Could you check a few things on this model? Use its own coordinates, in mm. Face numbers are marked on the shaded views. A direction names the side the tool comes from. Give positions to 0.01 mm unless a question says otherwise; leave off trailing zeros. Order: outer loops, then holes, each group sorted by start corner. A loop starts at its lowest first (then second) coordinate and runs counter-clockwise, first axis right, second up. Notation, with made-up numbers: M 53,87.5 L 100,87.5 A30 ccw 100,111.5 Z; hole C 29,52.5 d5. An arc over 180 degrees is marked long. Answer in a Markdown table with one row per item. Add a question column.
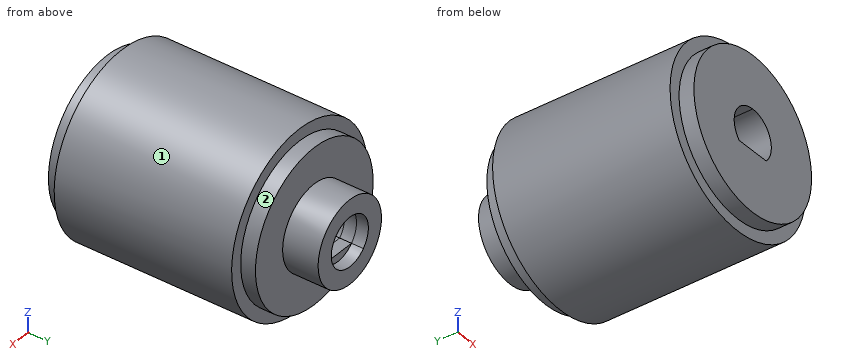
```python
from build123d import *
from build123d.topology import SkipClean

# Parameters (mm, degrees)
SKETCH1_R           = 15
BOSS_EXTRUDE1_DEPTH = 60
CUT_EXTRUDE1_START  = -2.5
SKETCH2_R           = 15
SKETCH2_R_2         = 13
CUT_EXTRUDE1_DEPTH  = 2.5
SKETCH3_R           = 15
CUT_EXTRUDE2_DEPTH  = 25
SKETCH4_R           = 15
SKETCH4_R_2         = 13
CUT_EXTRUDE3_DEPTH  = 2.5
SKETCH6_R           = 2.870458913
BOSS_EXTRUDE2_DEPTH = 9.5
SKETCH7_R           = 7
BOSS_EXTRUDE3_DEPTH = 2
SKETCH8_R           = 19
CUT_EXTRUDE4_DEPTH  = 43.649736224
CUT_EXTRUDE5_DEPTH  = 43.649736224
SKETCH10_R          = 7
BOSS_EXTRUDE4_DEPTH = 2
CUT_EXTRUDE6_DEPTH  = 45.395945761
SKETCH12_R          = 7
BOSS_EXTRUDE5_DEPTH = 2
CUT_EXTRUDE7_DEPTH  = 47.16275555
CUT_EXTRUDE8_START  = -2
SKETCH14_R          = 4.1
CUT_EXTRUDE8_DEPTH  = 2


with BuildPart() as part:
    # Sketch1 → Boss-Extrude1 (new body)
    with BuildSketch(Plane(origin=(0, 0, 0), x_dir=(1, 0, 0), z_dir=(0, 1, 0))):
        with Locations(Location((0, 0, 0), (0, 0, 270))):
            Circle(SKETCH1_R)
    extrude(amount=BOSS_EXTRUDE1_DEPTH)

    # Sketch2 → Cut-Extrude1 (cut)
    with BuildSketch(Plane(origin=(0, 60, 0), x_dir=(1, 0, 0), z_dir=(0, 1, 0)).offset(CUT_EXTRUDE1_START)):
        with Locations(Location((0, 0, 0), (0, 0, 270))):
            Circle(SKETCH2_R)
        with Locations(Location((0, 0, 0), (0, 0, 270))):
            Circle(SKETCH2_R_2, mode=Mode.SUBTRACT)
    extrude(amount=CUT_EXTRUDE1_DEPTH, mode=Mode.SUBTRACT)

    # Sketch3 → Cut-Extrude2 (cut)
    with BuildSketch(Plane.XZ):
        with Locations(Location((0, 0, 0), (0, 0, 270))):
            Circle(SKETCH3_R)
    extrude(amount=-CUT_EXTRUDE2_DEPTH, mode=Mode.SUBTRACT)

    # Sketch4 → Cut-Extrude3 (cut)
    with BuildSketch(Plane.XZ.offset(-25)):
        with Locations(Location((0, 0, 0), (0, 0, 270))):
            Circle(SKETCH4_R)
        with Locations(Location((0, 0, 0), (0, 0, 90))):
            Circle(SKETCH4_R_2, mode=Mode.SUBTRACT)
    extrude(amount=-CUT_EXTRUDE3_DEPTH, mode=Mode.SUBTRACT)

    # Sketch6 → Boss-Extrude2 (add)
    with BuildSketch(Plane.XZ.offset(-25)):
        with Locations(Location((0, 0, 0), (0, 0, 270))):
            Circle(SKETCH6_R)
    extrude(amount=BOSS_EXTRUDE2_DEPTH)

    # Sketch7 → Boss-Extrude3 (add)
    with BuildSketch(Plane(origin=(0, 60, 0), x_dir=(1, 0, 0), z_dir=(0, 1, 0))):
        with Locations(Location((0, 0, 0), (0, 0, 270))):
            Circle(SKETCH7_R)
    extrude(amount=BOSS_EXTRUDE3_DEPTH)

    # Sketch8 → Cut-Extrude4 (cut, through all)
    with BuildSketch(Plane.XZ.offset(-25)):
        Circle(SKETCH8_R)
    extrude(amount=CUT_EXTRUDE4_DEPTH, mode=Mode.SUBTRACT)

    # Sketch9 → Cut-Extrude5 (cut, through all)
    with BuildSketch(Plane(origin=(0, 62, 0), x_dir=(1, 0, 0), z_dir=(0, 1, 0))):
        with BuildLine():
            ThreePointArc((-2.994995826, 2.8), (-3.760983914, -1.632482772), (0, -4.1))
            Line((0, -4.1), (0, 2.8))
            Line((0, 2.8), (-2.994995826, 2.8))
        make_face()
        with BuildLine():
            Line((0, 2.8), (0, -4.1))
            ThreePointArc((0, -4.1), (3.760983914, -1.632482772), (2.994995826, 2.8))
            Line((2.994995826, 2.8), (0, 2.8))
        make_face()
    extrude(amount=-CUT_EXTRUDE5_DEPTH, mode=Mode.SUBTRACT)

    # Sketch10 → Boss-Extrude4 (add)
    with BuildSketch(Plane(origin=(0, 62, 0), x_dir=(1, 0, 0), z_dir=(0, 1, 0))):
        with Locations(Location((0, 0, 0), (0, 0, 270))):
            Circle(SKETCH10_R)
    extrude(amount=BOSS_EXTRUDE4_DEPTH)

    # Sketch11 → Cut-Extrude6 (cut, through all)
    with SkipClean():  # the faces are left unmerged after this step: merging them gives an invalid solid
        with BuildSketch(Plane.XZ.offset(-25)):
            with BuildLine():
                Line((-2.994995826, -2.8), (2.994995826, -2.8))
                ThreePointArc((2.994995826, -2.8), (0, 4.1), (-2.994995826, -2.8))
            make_face()
        extrude(amount=-CUT_EXTRUDE6_DEPTH, mode=Mode.SUBTRACT)

    # Sketch12 → Boss-Extrude5 (add)
    with SkipClean():  # the faces are left unmerged after this step: merging them gives an invalid solid
        with BuildSketch(Plane(origin=(0, 64, 0), x_dir=(1, 0, 0), z_dir=(0, 1, 0))):
            with Locations(Location((0, 0, 0), (0, 0, 270))):
                Circle(SKETCH12_R)
        extrude(amount=BOSS_EXTRUDE5_DEPTH)

    # Sketch13 → Cut-Extrude7 (cut, through all)
    with SkipClean():  # the faces are left unmerged after this step: merging them gives an invalid solid
        with BuildSketch(Plane.XZ.offset(-25)):
            with BuildLine():
                Line((-2.994995826, -2.8), (2.994995826, -2.8))
                ThreePointArc((2.994995826, -2.8), (0, 4.1), (-2.994995826, -2.8))
            make_face()
        extrude(amount=-CUT_EXTRUDE7_DEPTH, mode=Mode.SUBTRACT)

    # Sketch14 → Cut-Extrude8 (cut)
    with SkipClean():  # the faces are left unmerged after this step: merging them gives an invalid solid
        with BuildSketch(Plane(origin=(0, 66, 0), x_dir=(1, 0, 0), z_dir=(0, 1, 0)).offset(CUT_EXTRUDE8_START)):
            with Locations(Location((0, 0, 0), (0, 0, 136.927218653))):
                Circle(SKETCH14_R)
        extrude(amount=CUT_EXTRUDE8_DEPTH, mode=Mode.SUBTRACT)


solid = part.part
```
1. Suppose I cut it at B-B on x = -1. List the corners of the cut face in (y, z) for me, plus the area to 3 significant figures.
2. Will these pins go through, and if not, where does the flat tip stop? P1, Ø2, axis at x = -10, y = 50, coming from the -Z side; P2, Ø9.5, axis at x = 0, z = 0, coming from the -Y side; P3, Ø10, axis at x = -7, z = 10, coming from the +Y side; P4, Ø2, axis at y = 29.5, z = -3, coming from the -X side.
3. Suppose I cut it at D-D on y = 38.5. List the corners of the cut face in (x, z) for me (3 decimals), plus the area to 3 significant figures.
4. If I drill on line 1 along X through (y, z) = (63.4, 0); line 2 along Y through (x, z) = (-6.25, -11.75); line 3 along Y through (x, z) = (-7.5, -2), over which ranges is the centre line in solid material (lowest first)? Write a range as [from, to].
5. Suppose I cut it at A-A on z = 0. List the corners of the cut face in (x, y) for me, plus the area to 3 significant figures.
6. Suppose I cut it at C-C on x = -8. List the corners of the cut face in (y, z) for me.
7. For the marked faces 1 and 2, which set-ups out of +Z, -Z, +X, -X, +Y, -Y let a thin tool reach every point of the face, with its end or its side?
Findings below:
| question | item | result |
|---|---|---|
| 1 | outline | M 25,-12.96 L 27.5,-12.96 L 27.5,-14.97 L 57.5,-14.97 L 57.5,-12.96 L 60,-12.96 L 60,-6.93 L 66,-6.93 L 66,-3.98 L 64,-3.98 L 64,-2.8 L 25,-2.8 Z; M 25,3.98 L 66,3.98 L 66,6.93 L 60,6.93 L 60,12.96 L 57.5,12.96 L 57.5,14.97 L 27.5,14.97 L 27.5,12.96 L 25,12.96 Z |
| 1 | area | 831 mm2 |
| 2 | P1 | z = -12 |
| 2 | P2 | y = 25 |
| 2 | P3 | y = 60 |
| 2 | P4 | x = -14.87 |
| 3 | outline | C 0,0 d30; hole M -2.995,-2.8 L 2.995,-2.8 A4.1 ccw long Z |
| 3 | area | 659 mm2 |
| 4 | line 1 | [-7, -4.1], [4.1, 7] |
| 4 | line 2 | [27.5, 57.5] |
| 4 | line 3 | [25, 60] |
| 5 | outline | M -15,27.5 L -13,27.5 L -13,25 L -4.1,25 L -4.1,66 L -7,66 L -7,60 L -13,60 L -13,57.5 L -15,57.5 Z; M 4.1,25 L 13,25 L 13,27.5 L 15,27.5 L 15,57.5 L 13,57.5 L 13,60 L 7,60 L 7,66 L 4.1,66 Z |
| 5 | area | 778 mm2 |
| 6 | outline | M 25,-10.25 L 27.5,-10.25 L 27.5,-12.69 L 57.5,-12.69 L 57.5,-10.25 L 60,-10.25 L 60,10.25 L 57.5,10.25 L 57.5,12.69 L 27.5,12.69 L 27.5,10.25 L 25,10.25 Z |
| 7 | face 1 | +Y, -Y |
| 7 | face 2 | +Y |
